from build123d import *

# Parameters (mm, degrees)
SKETCH1_W           = 29.53979912
SKETCH1_H           = 15.405724453
BOSS_EXTRUDE1_DEPTH = 17
SKETCH3_W           = 1
SKETCH3_H           = 3.5
CUT_EXTRUDE2_DEPTH  = 2


# Read off the part's stored shape, not the designer's step: Cavity1
with BuildPart() as part:
    # Sketch1 → Boss-Extrude1 (new body)
    with BuildSketch(Plane.XY):
        with Locations((7.049151698, 0.989576641)):
            Rectangle(SKETCH1_W, SKETCH1_H)
    extrude(amount=BOSS_EXTRUDE1_DEPTH)

    # Cavity1 outline → Cavity1 (revolve, cut)
    with BuildSketch(Plane(origin=(7.02830498, 0, 0), x_dir=(1, 0, 0), z_dir=(0, 0, 1))):
        Polygon((13.126805589, -4), (7.414213562, 0), (13.414213562, 6), (13.414213562, 8), (0, 8), (0, -6), (13.126805589, -6), align=None)
    revolve(axis=Axis((7.02830498, 0, 0), (0, 1, 0)), mode=Mode.SUBTRACT)

    # Sketch3 → Cut-Extrude2 (cut)
    with BuildSketch(Plane(origin=(0, 0, 0), x_dir=(-1, 0, 0), z_dir=(0, 0, -1))):
        with Locations((-19.819051258, 0.597141886)):
            Rectangle(SKETCH3_W, SKETCH3_H)
        with Locations((5.720747862, 0.597141886)):
            Rectangle(SKETCH3_W, SKETCH3_H)
    extrude(amount=-CUT_EXTRUDE2_DEPTH, mode=Mode.SUBTRACT)


solid = part.part
Can you work these out from the model? Positions are in its coordinate system, mm. A direction names the side the tool comes from. Coordinates: 2 decimals unless noted, no trailing zeros. Write each loop counter-clockwise with the first axis right and the second up, starting at its lowest first coordinate (ties: lowest second). Pieces come first, ordered by that corner, then holes. Notation, with made-up numbers: (-21, -8) - (20, -8) arc R18 cw to (20, 16) - close; hole circle Ø2 at (77, -29). An arc over 180 degrees is marked (long way). Return JSON: item names as keys, results as strings. Group by question number.
Item 1: We'd pull the mould along X, two halves only. Please class faces 3 (the face through (7, -6, 5)), 4 (the face through (9.2, -6.4, 0)), 5 (the face through (21.819, 1, 8)): pulls with the +X half, pulls with the -X half, needs draft (parallel to the pull), parting line crosses it, or undercut.
Item 2: If we section it at C-C (y = -5): Write out the boundary of the cut face in (x, z).
Item 3: Please list where these lines run through material, in increasing order: probe 1 along Y at (x, z) = (6.5, 7); probe 2 along Y at (x, z) = (2.5, 9.5); probe 3 along Y at (x, z) = (8.5, 12).
Item 4: If we section it at B-B (z = 8.75): Count the separate pieces of the cut face and the enclosed holes in it, then the cut area to 3 significant figures.
Item 5: Which directions (+Z, -Z, +X, -X, +Y, -Y) give clear straight access to the entire face, cutting with the end or side of a thin tool? Please do faces 1 (the face through (19.319, 1, 1)), 2 (the face through (7, 1, 17)).
Item 6: If we section it at A-A (y = 7.25): Write out the boundary of the cut face in (x, z), then the cut area to 3 significant figures.
Item 7: I'm going to push a flat-ended pin straight in: pin 1 Ø0.5 at (x, y) = (20, 0.5) entering from -Z. Where does the tip first touch, or does it pass through?
Return value:
{
 "1": {"face 3": "undercut", "face 4": "needs draft", "face 5": "pulls with the +X half"},
 "2": {"outline": "(-7.72, 0) - (-6.1, 0) arc R13.13 cw to (20.16, 0) - (21.82, 0) - (21.82, 17) - (-7.72, 17) - close"},
 "3": {"probe 1": "y = -6.71 to -6, 8 to 8.69", "probe 2": "y = -6.71 to -6, -2.18 to 3.11, 8 to 8.69", "probe 3": "y = -6.71 to -6, -3.27 to 4.68, 8 to 8.69"},
 "4": {"separate pieces": "1", "enclosed holes": "2", "area": "276 mm^2"},
 "5": {"face 1": "-Z", "face 2": "+Z, +X, -X, +Y, -Y"},
 "6": {"outline": "(-7.72, 0) - (-6.39, 0) arc R13.41 cw to (20.44, 0) - (21.82, 0) - (21.82, 17) - (-7.72, 17) - close", "area": "220 mm^2"},
 "7": {"pin 1": "stops at z = 2"}
}
